Source: three-view drawing plus pictorial views. Frame: mm from the lowest corner of the part. Give positions to 0.01 mm unless a question says otherwise; leave off trailing zeros. Loops run counter-clockwise (first coordinate to the right, second up) from the corner with the lowest first, then second, coordinate; pieces in that order, holes last. Notation, with made-up numbers: (30, 73.25) - (77, 73.25) arc R23 cw to (77, 99.25) - close; hole circle Ø11 at (5.5, 30.25). An arc over 180 degrees is marked (long way). Answer as a JSON object with one key per item and string values.
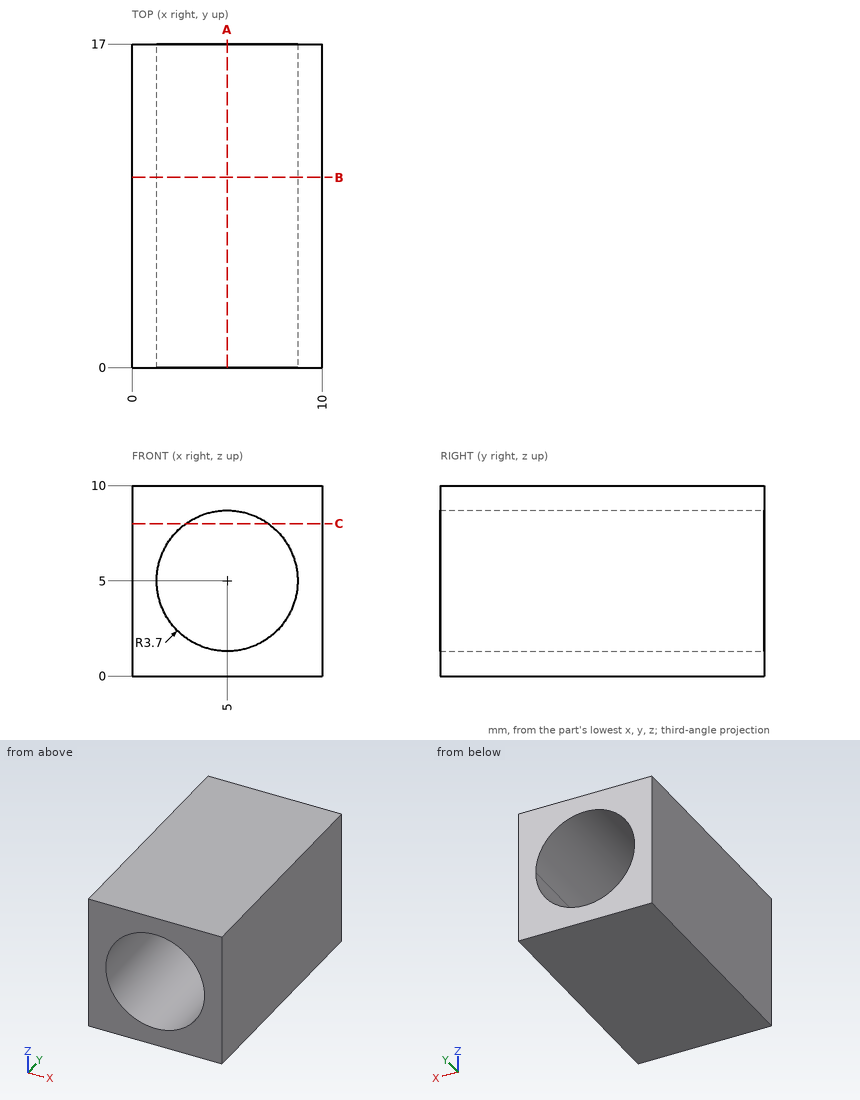
Item 1: Cut plane C-C (z = 8). Return loops of the section in (x, y).
Geometry check:
{"outline": "(0, 0) - (2.83, 0) - (2.83, 17) - (0, 17) - close; (7.17, 0) - (10, 0) - (10, 17) - (7.17, 17) - close"}
Item 2: Cut plane B-B (y = 10). Return loops of the section in (x, z).
Geometry check:
{"outline": "(0, 0) - (10, 0) - (10, 10) - (0, 10) - close; hole circle Ø7.4 at (5, 5)"}
Item 3: Material intervals for line 1 (X direction, y = 10.5, z = 5); line 2 (X direction, y = 16, z = 3.25); line 3 (Z direction, x = 2.25, y = 8), sorted ascending. Write a range as [from, to].
Geometry check:
{"line 1": "x = [0, 1.3], [8.7, 10]", "line 2": "x = [0, 1.74], [8.26, 10]", "line 3": "z = [0, 2.52], [7.48, 10]"}
Item 4: Cut plane A-A (x = 5). Return loops of the section in (y, z).
Geometry check:
{"outline": "(0, 0) - (17, 0) - (17, 1.3) - (0, 1.3) - close; (0, 8.7) - (17, 8.7) - (17, 10) - (0, 10) - close"}
